Geometry check sheet. Reference: the model listing, model coordinates, mm. Round coordinates to 2 decimals unless told otherwise and drop trailing zeros.
(1) Thickness scan on L1, parallel to Y at x = -28, z = 5; L2, parallel to Y at x = -21.5, z = 5; L3, parallel to X at y = 79.5, z = 4.25. Record the ranges inside material, lowest first.
(2) Draft check along Y on faces 1 (the face through (-27.6, 86.12, 3.13)), 2 (the face through (-19, 58, 6.35)), 3 (the face through (-1.91, 1.81, 3.22)). Enter one of: pulls with the +Y half, pulls with the -Y half, needs draft (parallel to the pull), parting line crosses it, or undercut.
(3) Gauge pin test, flat end, axial feed: P1, Ø1, axis at x = -4.5, z = 1, coming from the -Y side. Record the tip position at first contact, or that the pin passes through.
Autodesk Inventor part; units mm, degrees
ref_plane "YZ Plane" through (0, 0, 0) normal (1, 0, 0) x (0, 1, 0)
ref_plane "XZ Plane" through (0, 0, 0) normal (0, 1, 0) x (-1, 0, 0)
ref_plane "XY Plane" through (0, 0, 0) normal (0, 0, 1) x (1, 0, 0)
sketch "Sketch1" plane through (0, 0, 0) normal (0, 0, 1) x (1, 0, 0)
  line L0 (0, 0) -> (0, 114.3)
  line L1 (0, 0) -> (53.8815, 0) construction
  line L2 (0, 114.3) -> (76.2, 114.3) construction
  line L3 (0, 114.3) -> (-38.1, 114.3)
  line L4 (-38.1, 114.3) -> (-38.1, 0)
  line L5 (0, 0) -> (-38.1, 0)
  dimension "d0" = 114.3
  dimension "d86" = 38.1
extrude "Extrusion1" add sketch "Sketch1" along normal blind 6.35
fillet "Fillet1" radius 6.35 2 edges at (0, 114.3, 3.175) (0, 0, 3.175)
sketch "Sketch8" plane through (0, 0, 0) normal (0, 0, -1) x (-1, 0, 0)
  circle A0 centre (18.9128, 88.9) radius 2.54
  circle A1 centre (10.0465, 93.0252) radius 1.3589
  circle A2 centre (9.7264, 85.5476) radius 1.3589
  circle A3 centre (14.7876, 80.0337) radius 1.3589
  circle A4 centre (22.2652, 79.7136) radius 1.3589
  circle A5 centre (27.7791, 84.7748) radius 1.3589
  circle A6 centre (28.0992, 92.2524) radius 1.3589
  circle A7 centre (23.038, 97.7663) radius 1.3589
  circle A8 centre (15.5603, 98.0864) radius 1.3589
  line L0 (38.1, 0) -> (6.35, 0)
  point P0 (0, 0)
  dimension "d60" = 5.08
  dimension "d61" = 2.7178
  dimension "d62" = 9.779
  dimension "d65" = 360
  dimension "d87" = 88.9
extrude "Extrusion7" cut sketch "Sketch8" against normal blind 25.4 contours A1 | A2 | A3 | A4 | A5 | A6 | A7 | A8
sketch "Sketch9" plane through (0, 0, 6.35) normal (0, 0, 1) x (1, 0, 0)
  circle A0 centre (-23.038, 97.7663) radius 1.3589
  circle A1 centre (-14.7876, 80.0337) radius 1.3589
  circle A2 centre (-27.7791, 84.7748) radius 1.3589
  point P0 (0, 0)
  point P1 (-23.2077, 93.1949)
  dimension "d69" = 16.8402
  dimension "d70" = 8.4201
  dimension "d71" = 8.4201
properties part number "Triangle axle slide connector"
Found:
1. L1: y = 0 to 83.43, 86.12 to 90.9, 93.61 to 114.3
1. L2: y = 0 to 78.59, 80.84 to 114.3
1. L3: x = -38.1 to -23.61, -20.92 to -16.04, -13.54 to 0
2. face 1: undercut
2. face 2: needs draft
2. face 3: pulls with the -Y half
3. P1: stops at y = 0.15
